The model under review builds one solid part; all positions refer to its coordinate system, in mm. A direction names the side the tool comes from. Coordinates: 2 decimals unless noted, no trailing zeros. Write each loop counter-clockwise with the first axis right and the second up, starting at its lowest first coordinate (ties: lowest second). Pieces come first, ordered by that corner, then holes. Notation, with made-up numbers: (86.5, 9.5) -> (122.5, 9.5) arc R34 ccw to (122.5, 44.5) -> close; hole circle Ø4 at (-39.5, 10.5). An arc over 180 degrees is marked (long way). Put each result on its own line as item: value. Start each with the question number.
from build123d import *

# Parameters (mm, degrees)
F0_W      = 24.2
F0_H      = 34.3
F1_DEPTH  = 12
F2_W      = 20.1999982953
F2_H      = 30.2999982953
F3_DEPTH  = 10
F4_W      = 2.0000008523
F4_H      = 12
F5_DEPTH  = 10
F6_W      = 10.0999991477
F6_H      = 2.0000008523
F7_DEPTH  = 10
F8_W      = 24.2
F8_H      = 2.6
F9_DEPTH  = 5
F10_W     = 24.2
F10_H     = 2.6
F11_DEPTH = 3


with BuildPart() as f1:
    # F0 (on Top) → F1 (new body)
    with BuildSketch(Plane.XY):
        with Locations((12.1, 17.15)):
            Rectangle(F0_W, F0_H)
    extrude(amount=F1_DEPTH)

    # F2 (on face) → F3 (cut)
    with BuildSketch(Plane.XY.offset(12)):
        with Locations((12.1, 17.15)):
            Rectangle(F2_W, F2_H)
    extrude(amount=-F3_DEPTH, mode=Mode.SUBTRACT)

    # F4 (on face) → F5 (cut)
    with BuildSketch(Plane.XY.offset(12)):
        with Locations((1.0000004262, 8.0000008523)):
            Rectangle(F4_W, F4_H)
    extrude(amount=-F5_DEPTH, mode=Mode.SUBTRACT)

    # F6 (on face) → F7 (cut)
    with BuildSketch(Plane.XY.offset(12)):
        with Locations((7.0500004262, 33.2999995738)):
            Rectangle(F6_W, F6_H)
    extrude(amount=-F7_DEPTH, mode=Mode.SUBTRACT)

    # F8 (on face) → F9 (cut)
    with BuildSketch(Plane.XY.offset(12)):
        with Locations((12.1, 27.7652371407)):
            Rectangle(F8_W, F8_H)
    extrude(amount=-F9_DEPTH, mode=Mode.SUBTRACT)

    # F10 (on face) → F11 (cut)
    with BuildSketch(Plane.XY.offset(12)):
        with Locations((12.1, 21.0815354913)):
            Rectangle(F10_W, F10_H)
    extrude(amount=-F11_DEPTH, mode=Mode.SUBTRACT)


solid = f1.part
1. Consider section D-D on x = 18.75. State the section outline as (y, z) points, then the cut area to 3 significant figures.
2. Consider section C-C on y = 28. State the section outline as (x, z) points, then the cut area to 3 significant figures.
3. The part is to be moulded in two halves that separate along Y. For faces 1 (the flat face through (15, 34.3, 5)), 2 (the flat face through (12, 17, 0)), 3 (the flat face through (23, 21, 9)), 4 (the flat face through (1, 22.382, 11)), say which applies: released by +Y, released by -Y, zero draft, split by the parting line, or undercut.
4. Consider section B-B on z = 8. State the section outline as (x, y) points, then the cut area to 3 significant figures.
5. Tool access review of faces 5 (the flat face through (23, 19.782, 11)), 6 (the flat face through (0, 21, 5)), 7 (the flat face through (17, 1, 12)), 8 (the flat face through (11, 2, 7)), 9 (the flat face through (22.2, 17, 7)): name each direction out of +Z, -Z, +X, -X, +Y, -Y from which nothing blocks a thin tool from reaching the whole face with its end or side.
6. Insertion check: P1, Ø1, axis at x = 22.5, y = 21.5, coming from the +Z side; P2, Ø0.6, axis at x = 1, y = 27.5, coming from the +Z side; P3, Ø1, axis at x = 10, y = 16, coming from the +Z side. Each pin has a flat end and moves straight along its axis. Give the tip position at first contact, or say it passes through.
7. Wall thickness on line 1 (Y direction, x = 15, z = 10.75); line 2 (X direction, y = 33.5, z = 3.75); line 3 (X direction, y = 16, z = 3): over which ranges is each line inside the solid? List them lowest first. Write a range as from..to.
8. Consider section A-A on z = 3.75. State the section outline as (x, y) points, then the cut area to 3 significant figures.
Output values:
1. outline: (0, 0) -> (34.3, 0) -> (34.3, 12) -> (32.3, 12) -> (32.3, 2) -> (2, 2) -> (2, 12) -> (0, 12) -> close
1. area: 109 mm^2
2. outline: (0, 0) -> (24.2, 0) -> (24.2, 7) -> (22.2, 7) -> (22.2, 2) -> (2, 2) -> (2, 7) -> (0, 7) -> close
2. area: 68.4 mm^2
3. face 1: released by +Y
3. face 2: zero draft
3. face 3: undercut
3. face 4: undercut
4. outline: (0, 0) -> (24.2, 0) -> (24.2, 26.47) -> (22.2, 26.47) -> (22.2, 2) -> (0, 2) -> close; (0, 14) -> (2, 14) -> (2, 26.47) -> (0, 26.47) -> close; (0, 29.07) -> (2, 29.07) -> (2, 34.3) -> (0, 34.3) -> close; (12.1, 32.3) -> (22.2, 32.3) -> (22.2, 29.07) -> (24.2, 29.07) -> (24.2, 34.3) -> (12.1, 34.3) -> close
4. area: 163 mm^2
5. face 5: +Z, +X, -X
5. face 6: +Z, -Z, -X, +Y, -Y
5. face 7: +Z, +X, -X, +Y, -Y
5. face 8: +Z, -X
5. face 9: +Z
6. P1: stops at z = 9
6. P2: stops at z = 7
6. P3: stops at z = 2
7. line 1: y = 0..2, 32.3..34.3
7. line 2: x = 0..2, 12.1..24.2
7. line 3: x = 0..2, 22.2..24.2
8. outline: (0, 0) -> (24.2, 0) -> (24.2, 34.3) -> (12.1, 34.3) -> (12.1, 32.3) -> (22.2, 32.3) -> (22.2, 2) -> (0, 2) -> close; (0, 14) -> (2, 14) -> (2, 34.3) -> (0, 34.3) -> close
8. area: 174 mm^2
